from build123d import *

# Parameters (mm, degrees)
BOX_EXTRUDE_PART_DEPTH         = 110
BOX_EXTRUDE_PART_DEPTH_BACK    = 5
BOX_TOP_VIEW_W                 = 140
BOX_TOP_VIEW_H                 = 120
INNER_BOX_CUT_W                = 120
INNER_BOX_CUT_H                = 100
INNER_BOX_CUT_1_DEPTH          = 65
SCISSOR_CROSSSECTION_W         = 115
SCISSOR_CROSSSECTION_H         = 10
SCISSOR_CORSSSECTION_CUT_DEPTH = 10
SHAFT_LOCATION_R               = 7.5
SHAFT_LOCATION_CUT_DEPTH       = 40
SKETCH2_R                      = 14
BEARING_LOCATION_CUT1_DEPTH    = 10
SKETCH8_R                      = 9.5
BEARING_LOCATION_CUT2_DEPTH    = 35
M6_TAPPED_HOLE3_AT_2_COUNT     = 2
M6_TAPPED_HOLE3_AT_2_PITCH     = 85.14693183
EDGES_FILLET_R                 = 4


with BuildPart() as part:
    # Box_top_view → Box_extrude_part (new, two sides: drawn at the far end of the back side and taken through both)
    with BuildSketch(Plane(origin=(0, 0, 0), x_dir=(1, 0, 0), z_dir=(0, 1, 0)).offset(-BOX_EXTRUDE_PART_DEPTH_BACK)):
        Rectangle(BOX_TOP_VIEW_W, BOX_TOP_VIEW_H)
    extrude(amount=BOX_EXTRUDE_PART_DEPTH + BOX_EXTRUDE_PART_DEPTH_BACK)

    # Inner_box_cut → Inner_box_cut_1 (cut)
    with BuildSketch(Plane(origin=(0, 110, 0), x_dir=(1, 0, 0), z_dir=(0, 1, 0))):
        Rectangle(INNER_BOX_CUT_W, INNER_BOX_CUT_H)
    extrude(amount=-INNER_BOX_CUT_1_DEPTH, mode=Mode.SUBTRACT)

    # Scissor_crossSection → Scissor_corssSection_cut (cut)
    with BuildSketch(Plane.XY.offset(60)):
        with Locations((0, 60)):
            Rectangle(SCISSOR_CROSSSECTION_W, SCISSOR_CROSSSECTION_H)
    extrude(amount=-SCISSOR_CORSSSECTION_CUT_DEPTH, mode=Mode.SUBTRACT)

    # Shaft_location → Shaft_location_cut (cut)
    with BuildSketch(Plane(origin=(0, 45, 0), x_dir=(1, 0, 0), z_dir=(0, 1, 0))):
        with Locations(Location((15, 0, 0), (0, 0, 270))):
            Circle(SHAFT_LOCATION_R)
        with Locations(Location((-15, 0, 0), (0, 0, 90))):
            Circle(SHAFT_LOCATION_R)
    extrude(amount=-SHAFT_LOCATION_CUT_DEPTH, mode=Mode.SUBTRACT)

    # Sketch2 → Bearing_location_cut1 (cut)
    with BuildSketch(Plane(origin=(0, 45, 0), x_dir=(1, 0, 0), z_dir=(0, 1, 0))):
        with Locations(Location((-15, 0, 0), (0, 0, 270))):
            Circle(SKETCH2_R)
        with Locations(Location((15, 0, 0), (0, 0, 90))):
            Circle(SKETCH2_R)
    extrude(amount=-BEARING_LOCATION_CUT1_DEPTH, mode=Mode.SUBTRACT)

    # Sketch8 → Bearing_location_cut2 (cut)
    with BuildSketch(Plane(origin=(0, 45, 0), x_dir=(1, 0, 0), z_dir=(0, 1, 0))):
        with Locations(Location((-15, 0, 0), (0, 0, 270))):
            Circle(SKETCH8_R)
    extrude(amount=-BEARING_LOCATION_CUT2_DEPTH, mode=Mode.SUBTRACT)

    # Sketch7 → M6 Tapped Hole3 (revolve, cut)
    with BuildSketch(Plane(origin=(0, 110, -55), x_dir=(0, 0, 1), z_dir=(1, 0, 0))):
        Polygon((0, 0), (0, 14.502151548), (2.5, 13), (2.5, 0.525), (3.025, 0), align=None)
    m6_tapped_hole3 = revolve(axis=Axis((0, 116.35, -55), (0, -1, 0)), mode=Mode.SUBTRACT)

    # M6 Tapped Hole3 at 2: M6 Tapped Hole3 ×2
    with Locations(*[Vector(-0.7633862853691146, 0, 0.645942241466174) * (i * M6_TAPPED_HOLE3_AT_2_PITCH) for i in range(1, M6_TAPPED_HOLE3_AT_2_COUNT)]):
        add(m6_tapped_hole3, mode=Mode.SUBTRACT)

    # M6_hole_mirror: M6 Tapped Hole3 across plane
    add(m6_tapped_hole3.mirror(Plane(origin=(0, 0, 0), x_dir=(0, 0, 1), z_dir=(1, 0, 0))), mode=Mode.SUBTRACT)

    # M6_hole_mirror copy 1 sketch → M6_hole_mirror copy 1 (revolve, cut)
    with BuildSketch(Plane(origin=(65, 110, 0), x_dir=(0, 0, 1), z_dir=(-1, 0, 0))):
        Polygon((0, 0), (0, -14.502151548), (2.5, -13), (2.5, -0.525), (3.025, 0), align=None)
    revolve(axis=Axis((65, 116.35, 0), (0, 1, 0)), mode=Mode.SUBTRACT)

    # M6_hole_mirror at the second plane: M6 Tapped Hole3 across plane
    add(m6_tapped_hole3.mirror(Plane.XY), mode=Mode.SUBTRACT)

    # M6_hole_mirror at the second plane copy → M6_hole_mirror at the second plane c 2 (revolve, cut)
    with BuildSketch(Plane(origin=(-65, 110, 0), x_dir=(0, 0, -1), z_dir=(1, 0, 0))):
        Polygon((0, 0), (0, -14.502151548), (2.5, -13), (2.5, -0.525), (3.025, 0), align=None)
    revolve(axis=Axis((-65, 116.35, 0), (0, 1, 0)), mode=Mode.SUBTRACT)

    # Edges_fillet
    edges_fillet_edges = [part.edges().sort_by_distance(p)[0] for p in [
        (70, -5, 0),
        (0, -5, -60),
        (-70, -5, 0),
        (-70, 52.5, -60),
        (70, 52.5, -60),
        (70, 52.5, 60),
        (-70, 52.5, 60),
        (0, -5, 60),
    ]]
    fillet(edges_fillet_edges, radius=EDGES_FILLET_R)


solid = part.part
Here's how the part is built. I have some questions about the finished solid (model axes, mm). A direction names the side the tool comes from. Give positions to 0.01 mm unless a question says otherwise; leave off trailing zeros. Loops run counter-clockwise (first coordinate to the right, second up) from the corner with the lowest first, then second, coordinate; pieces in that order, holes last. Notation, with made-up numbers: (80.25, -10) -> (116.25, -10) arc R8 ccw to (116.25, -2) -> close; hole circle Ø5 at (47.5, -6.5). An arc over 180 degrees is marked (long way). Answer as a JSON object with one key per item and string values. Group by question number.
Item 1: Will these pins go through, and if not, where does the flat tip stop? pin 1 (16.5 mm diameter, centred on x = -11.5, z = 3, fed in from +Y); pin 2 (8.5 mm diameter, centred on x = -13.5, z = -0.5, fed in from +Y).
Item 2: Thinking about a two-plate mould opening in X: for faces 4 (the flat face through (-24.1, 35, -3.3)), 5 (the flat face through (70, 54, 1)), 6 (the cylindrical face through (-68.859, 55.277, 58.797)), which applies, pulls with the +X half, pulls with the -X half, needs draft (parallel to the pull), parting line crosses it, or undercut?
Item 3: On a 3-axis mill with a long thin cutter (end or side, diameter ignored), from which of +Z, -Z, +X, -X, +Y, -Y can I reach the whole of each face in a straight line? I mean faces 1 (the flat face through (-1, 65, 55)), 2 (the flat face through (-1, 78, -50)), 3 (the cylindrical face through (68.859, 55.277, -58.797)). Say none if no direction works.
Item 4: Imagine slicing it at B-B on y = 99. Write out the boundary of the cut face in (x, z), then the cut area to 3 significant figures.
Item 5: Imagine slicing it at A-A on x = -35. Write out the boundary of the cut face in (y, z), then the cut area to 3 significant figures.
Item 6: I need wall thicknesses on L1, parallel to X at y = 39, z = 0; L2, parallel to X at y = 25, z = 0; L3, parallel to Z at x = 0, y = 105.25. Which ranges of each line are inside material? Lowest first, please.
Item 7: Imagine slicing it at D-D on x = 15. Write out the boundary of the cut face in (y, z).
Item 8: Imagine slicing it at C-C on z = -32. Write out the boundary of the cut face in (x, y).
Answer list:
{
 "1": {"pin 1": "stops at y = 35", "pin 2": "stops at y = 5"},
 "2": {"face 4": "undercut", "face 5": "pulls with the +X half", "face 6": "pulls with the -X half"},
 "3": {"face 1": "+Z", "face 2": "+Y", "face 3": "-Z, +X, +Y, -Y"},
 "4": {"outline": "(-70, -56) arc R4 ccw to (-66, -60) -> (66, -60) arc R4 ccw to (70, -56) -> (70, 56) arc R4 ccw to (66, 60) -> (-66, 60) arc R4 ccw to (-70, 56) -> close; hole circle Ø5 at (-65, 0); hole (-60, -50) -> (60, -50) -> (60, 50) -> (-60, 50) -> close; hole circle Ø5 at (0, -55); hole circle Ø5 at (0, 55); hole circle Ø5 at (65, 0)", "area": "4,710 mm2"},
 "5": {"outline": "(-5, -56) arc R4 ccw to (-1, -60) -> (110, -60) -> (110, -50) -> (45, -50) -> (45, 50) -> (55, 50) -> (55, 60) -> (-1, 60) arc R4 ccw to (-5, 56) -> close; (65, 50) -> (110, 50) -> (110, 60) -> (65, 60) -> close", "area": "7,190 mm2"},
 "6": {"L1": "x = -70 to -29, -1 to 1, 29 to 70", "L2": "x = -70 to -24.5, -5.5 to 7.5, 22.5 to 70", "L3": "z = -60 to -57.5, -52.5 to -50, 50 to 52.5, 57.5 to 60"},
 "7": {"outline": "(-5, -56) arc R4 ccw to (-1, -60) -> (110, -60) -> (110, -50) -> (45, -50) -> (45, -14) -> (35, -14) -> (35, -7.5) -> (5, -7.5) -> (5, 7.5) -> (35, 7.5) -> (35, 14) -> (45, 14) -> (45, 50) -> (55, 50) -> (55, 60) -> (-1, 60) arc R4 ccw to (-5, 56) -> close; (65, 50) -> (110, 50) -> (110, 60) -> (65, 60) -> close"},
 "8": {"outline": "(-70, -1) arc R4 ccw to (-66, -5) -> (66, -5) arc R4 ccw to (70, -1) -> (70, 110) -> (60, 110) -> (60, 45) -> (-60, 45) -> (-60, 110) -> (-70, 110) -> close"}
}
